Can you work these out from the model? Positions are in its coordinate system, mm. A direction names the side the tool comes from. Coordinates: 2 decimals unless noted, no trailing zeros. Order: outer loops, then holes, each group sorted by start corner. A loop starts at its lowest first (then second) coordinate and runs counter-clockwise, first axis right, second up. Notation, with made-up numbers: (39.5, -38) -> (80.5, -38) arc R16 ccw to (80.5, -17) -> close; hole circle Ø1 at (-30, -33.5). An arc over 180 degrees is marked (long way). Write item = value, one per line.
Autodesk Inventor part; units mm, degrees
ref_plane "YZ Plane" through (0, 0, 0) normal (1, 0, 0) x (0, 1, 0)
ref_plane "XZ Plane" through (0, 0, 0) normal (0, 1, 0) x (-1, 0, 0)
ref_plane "XY Plane" through (0, 0, 0) normal (0, 0, 1) x (1, 0, 0)
sketch "Skizze1" plane through (0, 0, 0) normal (1, 0, 0) x (0, 1, 0)
  line L0 (0, -6) -> (0, 5)
  line L1 (0, 5) -> (-2.4, 5)
  line L2 (-2.4, 5) -> (-2.4, -5.1102)
  line L3 (-2.4, -5.1102) -> (-18, -14.5)
  line L4 (-18, -14.5) -> (-16.9686, -16.2135)
  line L5 (-16.9686, -16.2135) -> (0, -6)
  point P0 (0, 0)
  point P1 (0, -0.5)
  dimension "d0" = 5
  dimension "d1" = 2.4
  dimension "d3" = 14
  dimension "d4" = 18
  dimension "d12" = 2
  dimension "d15" = 6
extrude "Extrusion1" add sketch "Skizze1" along normal mid plane 36
sketch "Skizze2" plane through (-18, -2.4, -5.1102) normal (0, -1, 0) x (1, 0, 0)
  line L0 (18, 14.3529) -> (18, -15.346) construction
  line L1 (31.6, 4.4475) -> (30.6627, 3.5102)
  line L2 (30.6627, 3.5102) -> (29.3373, 3.5102)
  line L3 (29.3373, 3.5102) -> (28.4, 4.4475)
  line L4 (28.4, 4.4475) -> (28.4, 5.773)
  line L5 (28.4, 5.773) -> (29.3373, 6.7102)
  line L6 (29.3373, 6.7102) -> (30.6627, 6.7102)
  line L7 (30.6627, 6.7102) -> (31.6, 5.773)
  line L8 (31.6, 5.773) -> (31.6, 4.4475)
  line L9 (7.6, 4.4475) -> (6.6627, 3.5102)
  line L10 (6.6627, 3.5102) -> (5.3373, 3.5102)
  line L11 (5.3373, 3.5102) -> (4.4, 4.4475)
  line L12 (4.4, 4.4475) -> (4.4, 5.773)
  line L13 (4.4, 5.773) -> (5.3373, 6.7102)
  line L14 (5.3373, 6.7102) -> (6.6627, 6.7102)
  line L15 (6.6627, 6.7102) -> (7.6, 5.773)
  line L16 (7.6, 5.773) -> (7.6, 4.4475)
  line L17 (-7.2, 5.1102) -> (43.2, 5.1102) construction
  point P0 (18, 5.1102)
  point P1 (30, 5.1102)
  point P2 (6, 5.1102)
  dimension "d8" = 3.2
  dimension "d9" = 24
extrude "Extrusion2" cut sketch "Skizze2" against normal through all
chamfer "Fase1" distance 2 angle 45 1 edges at (0, -2.4, -5.1102)
sketch "Skizze3" plane through (-18, -2.4, 5) normal (0, -1, 0) x (1, 0, 0)
  line L0 (36, -8.1102) -> (0, -8.1102)
  line L1 (36, 0) -> (36, -8.1102)
  line L2 (0, 0) -> (36, 0)
  line L3 (0, -8.1102) -> (0, 0)
  line L4 (29.3373, -3.4) -> (30.6627, -3.4)
  line L5 (30.6627, -3.4) -> (31.6, -4.3373)
  line L6 (31.6, -4.3373) -> (31.6, -5.6627)
  line L7 (31.6, -5.6627) -> (30.6627, -6.6)
  line L8 (30.6627, -6.6) -> (29.3373, -6.6)
  line L9 (29.3373, -6.6) -> (28.4, -5.6627)
  line L10 (28.4, -5.6627) -> (28.4, -4.3373)
  line L11 (28.4, -4.3373) -> (29.3373, -3.4)
  line L12 (5.3373, -3.4) -> (6.6627, -3.4)
  line L13 (6.6627, -3.4) -> (7.6, -4.3373)
  line L14 (7.6, -4.3373) -> (7.6, -5.6627)
  line L15 (7.6, -5.6627) -> (6.6627, -6.6)
  line L16 (6.6627, -6.6) -> (5.3373, -6.6)
  line L17 (5.3373, -6.6) -> (4.4, -5.6627)
  line L18 (4.4, -5.6627) -> (4.4, -4.3373)
  line L19 (4.4, -4.3373) -> (5.3373, -3.4)
  line L20 (31.2426, -2) -> (28.7574, -2)
  line L21 (28.7574, -2) -> (27, -3.7574)
  line L22 (27, -3.7574) -> (27, -6.2426)
  line L23 (27, -6.2426) -> (28.7574, -8)
  line L24 (28.7574, -8) -> (31.2426, -8)
  line L25 (31.2426, -8) -> (33, -6.2426)
  line L26 (33, -6.2426) -> (33, -3.7574)
  line L27 (33, -3.7574) -> (31.2426, -2)
  point P0 (18, -5)
  point P1 (28.2105, -7.4531)
  point P2 (31.7895, -7.4531)
  dimension "d19" = 6
extrude "Extrusion3" cut sketch "Skizze3" along normal mid plane 2.2 contours L27 L26 L25 L24 L23 L22 L21 L20
mirror "Spiegeln1" about plane through (0, 0, 0) normal (1, 0, 0) of "Extrusion3"
sketch "Skizze4" plane through (-18, -18, -14.5) normal (0, -0.5156973, 0.8567708) x (1, 0, 0)
  line L0 (0, 16.2079) -> (36, 16.2079)
  line L1 (0, 0) -> (0, 16.2079)
  line L2 (0, 0) -> (36, 0)
  line L3 (36, 16.2079) -> (36, 0)
  line L4 (18, 32.4901) -> (18, -6.446) construction
  line L5 (19, 0) -> (20, 1)
  line L6 (20, 1) -> (21, 0)
  line L7 (20, 1) -> (20, 0) construction
  point P0 (18, 22.8995)
  dimension "d22" = 1
  dimension "d23" = 1
extrude "Extrusion4" cut sketch "Skizze4" against normal through all contours L5 L6 L2
mirror "Spiegeln2" [suppressed]
properties part number "Dribblerdaempfer Flex" material "Gummi, Silikon"
Item 1: I'm going to push flat-ended pins straight in: P1, Ø2.5, axis at x = 2, z = 1, coming from the -Y side; P2, Ø10, axis at x = -8, y = -8.5, coming from the +Z side; P3, Ø2, axis at x = 6.5, z = -4, coming from the -Y side; P4, Ø4, axis at y = -7.5, z = -11, coming from the +X side. Where does each tip first touch, or does it pass through?
A:
P1 = -2.4
P2 = -5.06
P3 = -3.47
P4 = 18
Item 2: I want a section at B-B, the plane y = -8.75. Please give me the cut outline in (x, z).
A:
outline = (-18, -11.27) -> (18, -11.27) -> (18, -8.93) -> (-18, -8.93) -> close
Item 3: I want a section at C-C, the plane z = -5. Please give me the cut outline in (x, y).
A:
outline = (-18, -3.47) -> (18, -3.47) -> (18, 0) -> (-18, 0) -> close
Item 4: If I drill on probe 1 along Y at (x, z) = (-15.5, 2); probe 2 along Z at (x, y) = (7, -8); probe 3 along Z at (x, y) = (-8.5, -12.5), over which ranges is the centre line in solid material (lowest first)?
A:
probe_1 = -2.4 to 0
probe_2 = -10.82 to -8.48
probe_3 = -13.52 to -11.19
Item 5: For faces 3 (the flat face through (12, -2, -3)), 4 (the flat face through (0.25, -3.24, -4.6)), 5 (the flat face through (-13.14, -0.66, 1.12)), which set-ups out of +Z, -Z, +X, -X, +Y, -Y let a thin tool reach every point of the face, with its end or its side?
A:
face_3 = -Y
face_4 = +Z, +X, -X, -Y
face_5 = +Y, -Y
Item 6: I want a section at A-A, the plane x = -1. Please give me the cut outline in (y, z), plus the area to 3 significant figures.
A:
outline = (-18, -14.5) -> (-16.97, -16.21) -> (0, -6) -> (0, 5) -> (-2.4, 5) -> (-2.4, -3.11) -> (-4.11, -6.14) -> close
area = 65.1 mm2
Item 7: If we mould it in two halves opening along X, with no side actions, what happens to faces 1 (the flat face through (-0.252, -10.96, -10.262)), 2 (the flat face through (12, -2, 3))? For each: pulls with the +X half, pulls with the -X half, needs draft (parallel to the pull), parting line crosses it, or undercut.
A:
face_1 = needs draft
face_2 = undercut
